Autodesk Fusion 360 part; units mm, degrees
sketch "Sketch1" plane through (0, 0, 0) normal (0, 0, 1) x (1, 0, 0)
  line L0 (-17.126, 50.0374) -> (50, 50.0374)
  line L1 (50, 50.0374) -> (50, -9.4626)
  line L2 (50, -9.4626) -> (-17.126, -9.4626)
  line L3 (-17.126, -9.4626) -> (-17.126, 50.0374)
  circle A0 centre (-13.626, 46.5374) radius 1.75
  circle A1 centre (46.5, 46.5374) radius 1.75
  circle A2 centre (46.5, -5.9626) radius 1.75
  circle A3 centre (-13.626, -5.9626) radius 1.75
  line L4 (-17.1389, 39.0374) -> (3.0611, 39.0374)
  line L5 (3.0611, 39.0374) -> (3.0611, 19.5374)
  line L6 (3.0611, 19.5374) -> (-17.1389, 19.5374)
  line L7 (-17.1389, 19.5374) -> (-17.1389, 39.0374)
  line L8 (6.289, 16) -> (-8.711, 16)
  line L9 (-8.711, 16) -> (-8.711, 1)
  line L10 (-8.711, 1) -> (6.289, 1)
  line L11 (6.289, 1) -> (6.289, 16)
  line L12 (43.55, 43.4874) -> (8.95, 43.4874)
  line L13 (8.95, 43.4874) -> (8.95, -2.9126)
  line L14 (8.95, -2.9126) -> (43.55, -2.9126)
  line L15 (43.55, -2.9126) -> (43.55, 43.4874)
  dimension "d1" = 59.5
  dimension "d2" = 67.126
  dimension "d5" = 3.5
  dimension "d6" = 3.5
  dimension "d7" = 3.5
  dimension "d8" = 3.5
  dimension "d9" = 3.5
  dimension "d10" = 3.5
  dimension "d11" = 3.5
  dimension "d12" = 3.5
  dimension "d13" = 3.5
  dimension "d14" = 3.5
  dimension "d15" = 3.5
  dimension "d16" = 3.5
  dimension "d23" = 20.2
  dimension "d24" = 19.5
  dimension "d25" = 11
  dimension "d26" = 15
  dimension "d27" = 15
  dimension "d28" = 8.415
  dimension "d29" = 34.6
  dimension "d30" = 46.4
  dimension "d31" = 6.55
  dimension "d32" = 6.45
extrude "Extrude2" add sketch "Sketch1" along normal blind 2 contours L0 L1 L2 L3 L4 L5 L6
fillet "Fillet1" radius 2 4 edges at (50, -9.4626, 1) (-17.126, -9.4626, 1) (50, 50.0374, 1) (-17.126, 50.0374, 1)
extrude "Extrude3" add sketch "Sketch1" along normal blind 1 contours A0 | A1 | A2 | A3
Part model, mm, in its own coordinate system. A direction names the side the tool comes from. Coordinates: 2 decimals unless noted, no trailing zeros. Order: outer loops, then holes, each group sorted by start corner. A loop starts at its lowest first (then second) coordinate and runs counter-clockwise, first axis right, second up. Notation, with made-up numbers: (-36, 60) -> (9, 60) arc R23 cw to (9, 71) -> close; hole circle Ø4 at (83, 46.5). An arc over 180 degrees is marked (long way). Put each result on its own line as item: value. Start each with the question number.
(1) Pin check, flat tips, straight feed: pin 1 Ø3 at (x, y) = (-13.5, 46) entering from +Z; pin 2 Ø1 at (x, y) = (46.5, 47) entering from +Z; pin 3 Ø0.6 at (y, z) = (32.5, 1.5) entering from -X; pin 4 Ø12 at (x, y) = (16.5, 27.5) entering from +Z. Stop position of each tip, or through.
(2) Band-saw the part on A-A (x = -7). Give the cut face in (y, z), then the cut area to 3 significant figures.
(3) Probe line 1 along Y through (x, z) = (46.5, 1.65); line 2 along X through (y, z) = (15, 0.5); line 3 along Y through (x, z) = (9.5, 1.65). List the from-to ranges inside material, lowest first. Write a range as [from, to].
(4) Which spindle directions (+Z, -Z, +X, -X, +Y, -Y) get a long thin tool onto all of the face, cutting with end or side? Do faces 4 (the face through (-8.711, 9, 1)), 5 (the face through (-7, 39.037, 1)), 6 (the face through (48.117, -5.292, 1.493)). Say none if no direction does.
(5) Band-saw the part on B-B (y = 31). Give the cut face in (x, z), then the cut area to 3 significant figures.
(6) Band-saw the part on C-C (x = 5.5). Give the cut face in (y, z).
(7) Mould opens along Y. For faces 1 (the face through (16, 50.037, 1)), 2 (the face through (-14, -6, 1)), 3 (the face through (-17.126, 43, 1)) say: pulls with the +Y half, pulls with the -Y half, needs draft (parallel to the pull), parting line crosses it, or undercut.
(8) Band-saw the part on D-D (y = 11). Give the cut face in (x, z).
Determined:
1. pin 1: stops at z = 2
1. pin 2: stops at z = 1
1. pin 3: stops at x = 3.06
1. pin 4: passes through
2. outline: (-9.46, 0) -> (1, 0) -> (1, 2) -> (-9.46, 2) -> close; (16, 0) -> (19.54, 0) -> (19.54, 2) -> (16, 2) -> close; (39.04, 0) -> (50.04, 0) -> (50.04, 2) -> (39.04, 2) -> close
2. area: 50.0 mm²
3. line 1: y = [-9.46, -7.71], [-4.21, 44.79], [48.29, 50.04]
3. line 2: x = [-17.13, -8.71], [6.29, 8.95], [43.55, 50]
3. line 3: y = [-9.46, -2.91], [43.49, 50.04]
4. face 4: +Z, -Z
4. face 5: +Z, -Z, -X
4. face 6: +Z
5. outline: (3.06, 0) -> (8.95, 0) -> (8.95, 2) -> (3.06, 2) -> close; (43.55, 0) -> (50, 0) -> (50, 2) -> (43.55, 2) -> close
5. area: 24.7 mm²
6. outline: (-9.46, 0) -> (1, 0) -> (1, 2) -> (-9.46, 2) -> close; (16, 0) -> (50.04, 0) -> (50.04, 2) -> (16, 2) -> close
7. face 1: pulls with the +Y half
7. face 2: undercut
7. face 3: needs draft
8. outline: (-17.13, 0) -> (-8.71, 0) -> (-8.71, 2) -> (-17.13, 2) -> close; (6.29, 0) -> (8.95, 0) -> (8.95, 2) -> (6.29, 2) -> close; (43.55, 0) -> (50, 0) -> (50, 2) -> (43.55, 2) -> close
